from build123d import *

# Parameters (mm, degrees)
SKETCH2_W                  = 254
SKETCH2_H                  = 101.6
RECTANGLE_EXTRUSION_DEPTH  = 12.7
SKETCH4_W                  = 12.7
SKETCH4_H                  = 12.7
FRONT_FACE_TABS_DEPTH      = 12.7
SKETCH6_R                  = 2.24536
TAB_CURVE_FRONT_BACK_DEPTH = 12.7
SKETCH7_W                  = 12.7
SKETCH7_H                  = 12.7
RIGHT_FACE_TABS_DEPTH      = 12.7
SKETCH8_R                  = 2.24536
TAB_CURVE_LEFT_RIGHT_DEPTH = 12.7
SKETCH9_R                  = 2.5527
CUT_EXTRUDE1_DEPTH         = 154.979316793


with BuildPart() as part:
    # Sketch2 → Rectangle Extrusion (new body)
    with BuildSketch(Plane(origin=(0, 0, 0), x_dir=(1, 0, 0), z_dir=(0, 1, 0))):
        Rectangle(SKETCH2_W, SKETCH2_H)
    extrude(amount=RECTANGLE_EXTRUSION_DEPTH)

    # Sketch4 → Front Face Tabs (add)
    with BuildSketch(Plane.XY.offset(50.8)):
        with Locations((-63.5, 6.35)):
            Rectangle(SKETCH4_W, SKETCH4_H)
        with Locations((63.5, 6.35)):
            Rectangle(SKETCH4_W, SKETCH4_H)
    front_face_tabs = extrude(amount=FRONT_FACE_TABS_DEPTH)

    # Mirror Rear Face Tabs: Front Face Tabs across plane
    add(front_face_tabs.mirror(Plane.XY))

    # Sketch6 → Tab Curve Front Back (cut)
    with BuildSketch(Plane(origin=(0, 12.7, 0), x_dir=(1, 0, 0), z_dir=(0, 1, 0))):
        with Locations((-71.4375, 52.3875)):
            Circle(SKETCH6_R)
        with Locations((-55.5625, 52.3875)):
            Circle(SKETCH6_R)
        with Locations((55.5625, 52.3875)):
            Circle(SKETCH6_R)
        with Locations((71.4375, 52.3875)):
            Circle(SKETCH6_R)
        with Locations((71.4375, -52.3875)):
            Circle(SKETCH6_R)
        with Locations((55.5625, -52.3875)):
            Circle(SKETCH6_R)
        with Locations((-55.5625, -52.3875)):
            Circle(SKETCH6_R)
        with Locations((-71.4375, -52.3875)):
            Circle(SKETCH6_R)
    extrude(amount=-TAB_CURVE_FRONT_BACK_DEPTH, mode=Mode.SUBTRACT)

    # Sketch7 → Right Face Tabs (add)
    with BuildSketch(Plane(origin=(127, 0, 0), x_dir=(0, 0, -1), z_dir=(1, 0, 0))):
        with Locations((-25.4, 6.35)):
            Rectangle(SKETCH7_W, SKETCH7_H)
        with Locations((25.4, 6.35)):
            Rectangle(SKETCH7_W, SKETCH7_H)
    right_face_tabs = extrude(amount=RIGHT_FACE_TABS_DEPTH)

    # Mirror Left Face Tabs: Right Face Tabs across plane
    add(right_face_tabs.mirror(Plane(origin=(0, 0, 0), x_dir=(0, 0, 1), z_dir=(1, 0, 0))))

    # Sketch8 → Tab Curve Left Right (cut)
    with BuildSketch(Plane(origin=(0, 12.7, 0), x_dir=(1, 0, 0), z_dir=(0, 1, 0))):
        with Locations((128.5875, 33.3375)):
            Circle(SKETCH8_R)
        with Locations((128.5875, 17.4625)):
            Circle(SKETCH8_R)
        with Locations((128.5875, -17.4625)):
            Circle(SKETCH8_R)
        with Locations((128.5875, -33.3375)):
            Circle(SKETCH8_R)
        with Locations((-128.5875, -33.3375)):
            Circle(SKETCH8_R)
        with Locations((-128.5875, -17.4625)):
            Circle(SKETCH8_R)
        with Locations((-128.5875, 17.4625)):
            Circle(SKETCH8_R)
        with Locations((-128.5875, 33.3375)):
            Circle(SKETCH8_R)
    extrude(amount=-TAB_CURVE_LEFT_RIGHT_DEPTH, mode=Mode.SUBTRACT)

    # Sketch9 → Cut-Extrude1 (cut, through all)
    with BuildSketch(Plane.XZ):
        with Locations(Location((-107.95, 44.45, 0), (0, 0, 270))):
            Circle(SKETCH9_R)
        with Locations(Location((-120.65, 31.75, 0), (0, 0, 270))):
            Circle(SKETCH9_R)
        with Locations(Location((-120.65, 12.7, 0), (0, 0, 270))):
            Circle(SKETCH9_R)
        with Locations(Location((-120.65, -6.35, 0), (0, 0, 270))):
            Circle(SKETCH9_R)
        with Locations(Location((-120.65, -25.4, 0), (0, 0, 270))):
            Circle(SKETCH9_R)
        with Locations(Location((-88.9, 44.45, 0), (0, 0, 270))):
            Circle(SKETCH9_R)
        with Locations(Location((-69.85, 44.45, 0), (0, 0, 270))):
            Circle(SKETCH9_R)
        with Locations(Location((-50.8, 44.45, 0), (0, 0, 270))):
            Circle(SKETCH9_R)
        with Locations(Location((-31.75, 44.45, 0), (0, 0, 270))):
            Circle(SKETCH9_R)
        with Locations(Location((-12.7, 44.45, 0), (0, 0, 270))):
            Circle(SKETCH9_R)
        with Locations(Location((6.35, 44.45, 0), (0, 0, 270))):
            Circle(SKETCH9_R)
        with Locations(Location((25.4, 44.45, 0), (0, 0, 270))):
            Circle(SKETCH9_R)
        with Locations(Location((44.45, 44.45, 0), (0, 0, 270))):
            Circle(SKETCH9_R)
        with Locations(Location((63.5, 44.45, 0), (0, 0, 270))):
            Circle(SKETCH9_R)
        with Locations(Location((82.55, 44.45, 0), (0, 0, 270))):
            Circle(SKETCH9_R)
        with Locations(Location((101.6, 44.45, 0), (0, 0, 270))):
            Circle(SKETCH9_R)
        with Locations(Location((101.6, -44.45, 0), (0, 0, 90))):
            Circle(SKETCH9_R)
        with Locations(Location((82.55, -44.45, 0), (0, 0, 90))):
            Circle(SKETCH9_R)
        with Locations(Location((63.5, -44.45, 0), (0, 0, 90))):
            Circle(SKETCH9_R)
        with Locations(Location((44.45, -44.45, 0), (0, 0, 90))):
            Circle(SKETCH9_R)
        with Locations(Location((25.4, -44.45, 0), (0, 0, 90))):
            Circle(SKETCH9_R)
        with Locations(Location((6.35, -44.45, 0), (0, 0, 90))):
            Circle(SKETCH9_R)
        with Locations(Location((-12.7, -44.45, 0), (0, 0, 90))):
            Circle(SKETCH9_R)
        with Locations(Location((-31.75, -44.45, 0), (0, 0, 90))):
            Circle(SKETCH9_R)
        with Locations(Location((-50.8, -44.45, 0), (0, 0, 90))):
            Circle(SKETCH9_R)
        with Locations(Location((-69.85, -44.45, 0), (0, 0, 90))):
            Circle(SKETCH9_R)
        with Locations(Location((-88.9, -44.45, 0), (0, 0, 90))):
            Circle(SKETCH9_R)
        with Locations(Location((-107.95, -44.45, 0), (0, 0, 90))):
            Circle(SKETCH9_R)
        with Locations(Location((120.65, -25.4, 0), (0, 0, 90))):
            Circle(SKETCH9_R)
        with Locations(Location((120.65, -6.35, 0), (0, 0, 90))):
            Circle(SKETCH9_R)
        with Locations(Location((120.65, 12.7, 0), (0, 0, 90))):
            Circle(SKETCH9_R)
        with Locations(Location((120.65, 31.75, 0), (0, 0, 90))):
            Circle(SKETCH9_R)
    extrude(amount=-CUT_EXTRUDE1_DEPTH, mode=Mode.SUBTRACT)


solid = part.part
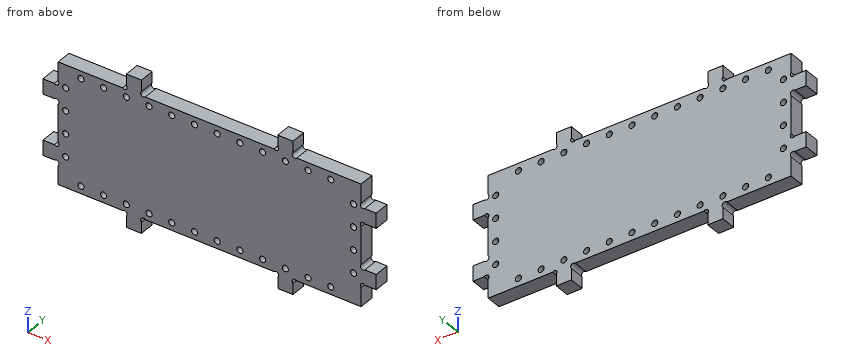
For this review, take the finished solid that the model builds, in its own axes (mm). Round coordinates to 2 decimals unless told otherwise and drop trailing zeros. Loops run counter-clockwise (first coordinate to the right, second up) from the corner with the lowest first, then second, coordinate; pieces in that order, holes last. Notation, with made-up numbers: (-29, 36.25) - (9, 36.25) arc R21 ccw to (9, 42.25) - close; hole circle Ø6 at (-3, 79). An arc over 180 degrees is marked (long way). Use one line per item in the form item = value.
1) Wall thickness on probe 1 along X at (y, z) = (10, -25.4); probe 2 along X at (y, z) = (7, -6.35); probe 3 along Z at (x, y) = (82.5, 5): over which ranges is each line inside the solid? List them lowest first.
Solutions:
probe_1 = -139.7 to -123.2, -118.1 to 118.1, 123.2 to 139.7
probe_2 = -127 to -123.2, -118.1 to 118.1, 123.2 to 127
probe_3 = -50.8 to -47, -41.9 to 41.9, 47 to 50.8
2) We need section B-B on z = -44.45. State how many separate pieces and enclosed holes the cut face has, then the cut area to 3 significant figures.
Solutions:
separate_pieces = 13
enclosed_holes = 0
area = 2,450 mm2
3) We need section A-A on x = 44.45. Write out the cut boundary in (y, z), then the cut area to 3 significant figures.
Solutions:
outline = (0, -50.8) - (12.7, -50.8) - (12.7, -47) - (0, -47) - close; (0, -41.9) - (12.7, -41.9) - (12.7, 41.9) - (0, 41.9) - close; (0, 47) - (12.7, 47) - (12.7, 50.8) - (0, 50.8) - close
area = 1,160 mm2
4) Clearance check with flat-ended pins moving along their axes: P1, Ø4, axis at x = 101.6, z = 44.45, coming from the +Y side; P2, Ø3, axis at y = 3, z = 61, coming from the -X side; P3, Ø1.5, axis at x = 111, y = 7, coming from the -Z side; P4, Ø6, axis at y = 8, z = 4, coming from the -X side. State where each tip first meets the part, or that it passes through.
Solutions:
P1 = through
P2 = -69.85
P3 = -50.8
P4 = -127
5) We need section D-D on z = 0.5. Write out the cut boundary in (x, y).
Solutions:
outline = (-127, 0) - (127, 0) - (127, 12.7) - (-127, 12.7) - close
